```python
from build123d import *

# Parameters (mm, degrees)
SKETCH1_R           = 1.5875
BOSS_EXTRUDE1_DEPTH = 6.35


with BuildPart() as part:
    # Sketch1 → Boss-Extrude1 (new body)
    with BuildSketch(Plane.XY):
        Polygon((6.35, 349.25), (14.9225, 349.25), (14.9225, 355.6), (32.0675, 355.6), (32.0675, 349.25), (49.2125, 349.25), (49.2125, 355.6), (66.3575, 355.6), (66.3575, 349.25), (83.5025, 349.25), (83.5025, 355.6), (100.6475, 355.6), (100.6475, 349.25), (117.7925, 349.25), (117.7925, 355.6), (134.9375, 355.6), (134.9375, 349.25), (152.0825, 349.25), (152.0825, 355.6), (169.2275, 355.6), (169.2275, 349.25), (186.3725, 349.25), (186.3725, 355.6), (203.5175, 355.6), (203.5175, 349.25), (220.6625, 349.25), (220.6625, 355.6), (237.8075, 355.6), (237.8075, 349.25), (254.9525, 349.25), (254.9525, 355.6), (272.0975, 355.6), (272.0975, 349.25), (289.2425, 349.25), (289.2425, 355.6), (306.3875, 355.6), (306.3875, 349.25), (323.5325, 349.25), (323.5325, 355.6), (340.6775, 355.6), (340.6775, 349.25), (349.25, 349.25), (349.25, 340.6775), (355.6, 340.6775), (355.6, 323.5325), (349.25, 323.5325), (349.25, 306.3875), (355.6, 306.3875), (355.6, 289.2425), (349.25, 289.2425), (349.25, 272.0975), (355.6, 272.0975), (355.6, 254.9525), (349.25, 254.9525), (349.25, 237.8075), (355.6, 237.8075), (355.6, 220.6625), (349.25, 220.6625), (349.25, 203.5175), (355.6, 203.5175), (355.6, 186.3725), (349.25, 186.3725), (349.25, 169.2275), (355.6, 169.2275), (355.6, 152.0825), (349.25, 152.0825), (349.25, 134.9375), (355.6, 134.9375), (355.6, 117.7925), (349.25, 117.7925), (349.25, 100.6475), (355.6, 100.6475), (355.6, 83.5025), (349.25, 83.5025), (349.25, 66.3575), (355.6, 66.3575), (355.6, 49.2125), (349.25, 49.2125), (349.25, 32.0675), (355.6, 32.0675), (355.6, 14.9225), (349.25, 14.9225), (349.25, 6.35), (340.6775, 6.35), (340.6775, 0), (323.5325, 0), (323.5325, 6.35), (306.3875, 6.35), (306.3875, 0), (289.2425, 0), (289.2425, 6.35), (272.0975, 6.35), (272.0975, 0), (254.9525, 0), (254.9525, 6.35), (237.8075, 6.35), (237.8075, 0), (220.6625, 0), (220.6625, 6.35), (203.5175, 6.35), (203.5175, 0), (186.3725, 0), (186.3725, 6.35), (169.2275, 6.35), (169.2275, 0), (152.0825, 0), (152.0825, 6.35), (134.9375, 6.35), (134.9375, 0), (117.7925, 0), (117.7925, 6.35), (100.6475, 6.35), (100.6475, 0), (83.5025, 0), (83.5025, 6.35), (66.3575, 6.35), (66.3575, 0), (49.2125, 0), (49.2125, 6.35), (32.0675, 6.35), (32.0675, 0), (14.9225, 0), (14.9225, 6.35), (6.35, 6.35), (6.35, 14.9225), (0, 14.9225), (0, 32.0675), (6.35, 32.0675), (6.35, 49.2125), (0, 49.2125), (0, 66.3575), (6.35, 66.3575), (6.35, 83.5025), (0, 83.5025), (0, 100.6475), (6.35, 100.6475), (6.35, 117.7925), (0, 117.7925), (0, 134.9375), (6.35, 134.9375), (6.35, 152.0825), (0, 152.0825), (0, 169.2275), (6.35, 169.2275), (6.35, 186.3725), (0, 186.3725), (0, 203.5175), (6.35, 203.5175), (6.35, 220.6625), (0, 220.6625), (0, 237.8075), (6.35, 237.8075), (6.35, 254.9525), (0, 254.9525), (0, 272.0975), (6.35, 272.0975), (6.35, 289.2425), (0, 289.2425), (0, 306.3875), (6.35, 306.3875), (6.35, 323.5325), (0, 323.5325), (0, 340.6775), (6.35, 340.6775), align=None)
        with Locations((10.668, 344.932)):
            Circle(SKETCH1_R, mode=Mode.SUBTRACT)
        with Locations((344.932, 344.932)):
            Circle(SKETCH1_R, mode=Mode.SUBTRACT)
        with Locations((344.932, 10.668)):
            Circle(SKETCH1_R, mode=Mode.SUBTRACT)
        with Locations((10.668, 10.668)):
            Circle(SKETCH1_R, mode=Mode.SUBTRACT)
    extrude(amount=BOSS_EXTRUDE1_DEPTH)


solid = part.part
```
Here's how the part is built. I have some questions about the finished solid (model axes, mm). Give positions to 0.01 mm unless a question says otherwise; leave off trailing zeros. Write each loop counter-clockwise with the first axis right and the second up, starting at its lowest first coordinate (ties: lowest second). Pieces come first, ordered by that corner, then holes. Notation, with made-up numbers: (22, 7.5) -> (44, 7.5) arc R27 cw to (44, 33.5) -> close; hole circle Ø3 at (60, -24.75). An arc over 180 degrees is marked (long way). Write each question's results on one line, items separated by ' | '.
Item 1: Suppose I cut it at C-C on z = 3.25. Give the number of separate pieces and of enclosed holes in the cut face, plus the area to 3 significant figures.
Output:
separate pieces: 1 | enclosed holes: 4 | area: 122,000 mm^2
Item 2: If I drill on L1, parallel to X at y = 253, z = 0.5, over which ranges is the centre line in solid material (lowest first)?
Output:
L1: x = 6.35 to 349.25
Item 3: For pin 1 Ø1.5 at (x, z) = (80.5, 3) entering from +Y; pin 2 Ø3 at (y, z) = (40, 2) entering from -X; pin 3 Ø2 at (y, z) = (260.5, 4) entering from -X, each with a flat end and sliding along its axis, tell me the tip position at first contact or that it passes through.
Output:
pin 1: stops at y = 349.25 | pin 2: stops at x = 6.35 | pin 3: stops at x = 0
Item 4: Suppose I cut it at A-A on x = 77.5. Write out the boundary of the cut face in (y, z).
Output:
outline: (6.35, 0) -> (349.25, 0) -> (349.25, 6.35) -> (6.35, 6.35) -> close
